```python
from build123d import *

# Parameters (mm, degrees)
CYLINDER049_R             = 1.38
CYLINDER049_DEPTH         = 40
CYLINDER030_R             = 1.75
CYLINDER030_DEPTH         = 10
CYLINDER029_R             = 5
CYLINDER029_DEPTH         = 10
CYLINDER024_R             = 8.5
CYLINDER024_DEPTH         = 2
BOX014_W                  = 0.5
BOX014_H                  = 1
BOX014_DEPTH              = 5
ARRAY002_COUNT            = 12
BOX015_W                  = 0.5
BOX015_H                  = 1
BOX015_DEPTH              = 5
CYLINDER026_R             = 4.5
CYLINDER026_DEPTH         = 8
CYLINDER028_R             = 1.5
CYLINDER028_DEPTH         = 4
BOX016_W                  = 1
BOX016_H                  = 10
BOX016_DEPTH              = 30
CYLINDER027_R             = 3
CYLINDER027_DEPTH         = 30
CYLINDER025_R             = 13
CYLINDER025_DEPTH         = 10
FUSION006_ROLL_ANGLE      = 180
FUSION006_PLACEMENT_ANGLE = 150
CYLINDER023_R             = 1.5
CYLINDER023_DEPTH         = 5
CYLINDER022_R             = 1.5
CYLINDER022_DEPTH         = 5
CYLINDER021_R             = 1.5
CYLINDER021_DEPTH         = 5
CYLINDER020_R             = 1.5
CYLINDER020_DEPTH         = 5
BOX010_W                  = 4
BOX010_H                  = 36
BOX010_DEPTH              = 38
BOX011_W                  = 4
BOX011_H                  = 36
BOX011_DEPTH              = 38
BOX012_W                  = 10
BOX012_H                  = 36
BOX012_DEPTH              = 3
BOX013_W                  = 10
BOX013_H                  = 36
BOX013_DEPTH              = 3
BOX009_W                  = 50
BOX009_H                  = 36
BOX009_DEPTH              = 3
CHAMFER_SIZE              = 2
CHAMFER001_SIZE           = 1


with BuildPart() as cylinder049:
    # Cylinder049 → Cylinder049 (new body)
    with BuildSketch(Plane(origin=(38, 57, 59), x_dir=(1, 0, 0), z_dir=(0, 0, 1))):
        Circle(CYLINDER049_R)
    extrude(amount=CYLINDER049_DEPTH)


with BuildPart() as cylinder030:
    # Cylinder030 → Cylinder030 (new body)
    with BuildSketch(Plane(origin=(33.25, 47.5, 71), x_dir=(1, 0, 0), z_dir=(0, 0, 1))):
        Circle(CYLINDER030_R)
    extrude(amount=CYLINDER030_DEPTH)


with BuildPart() as cylinder029:
    # Cylinder029 → Cylinder029 (new body)
    with BuildSketch(Plane(origin=(41, 43, 71), x_dir=(1, 0, 0), z_dir=(0, 0, 1))):
        Circle(CYLINDER029_R)
    extrude(amount=CYLINDER029_DEPTH)


with BuildPart() as cylinder024:
    # Cylinder024 → Cylinder024 (new body)
    with BuildSketch(Plane.XY.offset(10)):
        Circle(CYLINDER024_R)
    extrude(amount=CYLINDER024_DEPTH)


with BuildPart() as pin_array002:
    # Box014 → Box014 (new body)
    with BuildSketch(Plane(origin=(11, -0.5, -5), x_dir=(1, 0, 0), z_dir=(0, 0, 1))):
        with Locations((0.25, 0.5)):
            Rectangle(BOX014_W, BOX014_H)
    extrude(amount=BOX014_DEPTH)

    # Array002: Pin array002 ×12 about axis
    array002_axis = Axis((0, 0, 0), (0, 0, 1))


with BuildPart() as pin_array002_1:
    add(pin_array002.part)
    for i in range(1, ARRAY002_COUNT):
        add(pin_array002.part.rotate(array002_axis, i * 360 / ARRAY002_COUNT))


with BuildPart() as pin_central002:
    # Box015 → Box015 (new body)
    with BuildSketch(Plane(origin=(3, -0.5, -5), x_dir=(1, 0, 0), z_dir=(0, 0, 1))):
        with Locations((0.25, 0.5)):
            Rectangle(BOX015_W, BOX015_H)
    extrude(amount=BOX015_DEPTH)


with BuildPart() as cylinder026:
    # Cylinder026 → Cylinder026 (new body)
    with BuildSketch(Plane.XY.offset(12)):
        Circle(CYLINDER026_R)
    extrude(amount=CYLINDER026_DEPTH)


with BuildPart() as cylinder028:
    # Cylinder028 → Cylinder028 (new body)
    with BuildSketch(Plane(origin=(9, 0, 10), x_dir=(1, 0, 0), z_dir=(0, 0, 1))):
        Circle(CYLINDER028_R)
    extrude(amount=CYLINDER028_DEPTH)


with BuildPart() as obj1:
    # Box016 → Box016 (new body)
    with BuildSketch(Plane(origin=(2, -5, 20), x_dir=(1, 0, 0), z_dir=(0, 0, 1))):
        with Locations((0.5, 5)):
            Rectangle(BOX016_W, BOX016_H)
    extrude(amount=BOX016_DEPTH)


with BuildPart() as obj2:
    # Cylinder027 → Cylinder027 (new body)
    with BuildSketch(Plane.XY.offset(20)):
        Circle(CYLINDER027_R)
    extrude(amount=CYLINDER027_DEPTH)

    # Cut010: cut obj1
    add(obj1.part, mode=Mode.SUBTRACT)


with BuildPart() as selector_taladro:
    # Cylinder025 → Cylinder025 (new body)
    with BuildSketch(Plane.XY):
        Circle(CYLINDER025_R)
    extrude(amount=CYLINDER025_DEPTH)

    # Fusion006: union Cylinder024, Pin array002, Pin central002, Cylinder026, Cylinder028, obj2
    add(cylinder024.part)
    add(pin_array002_1.part)
    add(pin_central002.part)
    add(cylinder026.part)
    add(cylinder028.part)
    add(obj2.part)


with BuildPart() as selector_taladro_1:
    # Fusion006 roll: moved
    add(selector_taladro.part.rotate(Axis((0, 0, 0), (1, 0, 0)), FUSION006_ROLL_ANGLE))


with BuildPart() as selector_taladro_2:
    # Fusion006 placement: moved
    add(selector_taladro_1.part.moved(Location((40.992958, 43.010908, 90))).rotate(Axis((40.992958, 43.010908, 90), (0, 0, 1)), FUSION006_PLACEMENT_ANGLE))


with BuildPart() as cylinder023:
    # Cylinder023 → Cylinder023 (new body)
    with BuildSketch(Plane(origin=(65.5, 54, 39), x_dir=(1, 0, 0), z_dir=(0, 0, 1))):
        Circle(CYLINDER023_R)
    extrude(amount=CYLINDER023_DEPTH)


with BuildPart() as cylinder022:
    # Cylinder022 → Cylinder022 (new body)
    with BuildSketch(Plane(origin=(65.5, 38, 39), x_dir=(1, 0, 0), z_dir=(0, 0, 1))):
        Circle(CYLINDER022_R)
    extrude(amount=CYLINDER022_DEPTH)


with BuildPart() as cylinder021:
    # Cylinder021 → Cylinder021 (new body)
    with BuildSketch(Plane(origin=(8.5, 54, 39), x_dir=(1, 0, 0), z_dir=(0, 0, 1))):
        Circle(CYLINDER021_R)
    extrude(amount=CYLINDER021_DEPTH)


with BuildPart() as cylinder020:
    # Cylinder020 → Cylinder020 (new body)
    with BuildSketch(Plane(origin=(8.5, 38, 39), x_dir=(1, 0, 0), z_dir=(0, 0, 1))):
        Circle(CYLINDER020_R)
    extrude(amount=CYLINDER020_DEPTH)


with BuildPart() as box010:
    # Box010 → Box010 (new body)
    with BuildSketch(Plane(origin=(12, 28, 40), x_dir=(1, 0, 0), z_dir=(0, 0, 1))):
        with Locations((2, 18)):
            Rectangle(BOX010_W, BOX010_H)
    extrude(amount=BOX010_DEPTH)


with BuildPart() as box011:
    # Box011 → Box011 (new body)
    with BuildSketch(Plane(origin=(58, 28, 40), x_dir=(1, 0, 0), z_dir=(0, 0, 1))):
        with Locations((2, 18)):
            Rectangle(BOX011_W, BOX011_H)
    extrude(amount=BOX011_DEPTH)


with BuildPart() as box012:
    # Box012 → Box012 (new body)
    with BuildSketch(Plane(origin=(6, 28, 40), x_dir=(1, 0, 0), z_dir=(0, 0, 1))):
        with Locations((5, 18)):
            Rectangle(BOX012_W, BOX012_H)
    extrude(amount=BOX012_DEPTH)


with BuildPart() as box013:
    # Box013 → Box013 (new body)
    with BuildSketch(Plane(origin=(58, 28, 40), x_dir=(1, 0, 0), z_dir=(0, 0, 1))):
        with Locations((5, 18)):
            Rectangle(BOX013_W, BOX013_H)
    extrude(amount=BOX013_DEPTH)


with BuildPart() as cut028:
    # Box009 → Box009 (new body)
    with BuildSketch(Plane(origin=(12, 28, 75), x_dir=(1, 0, 0), z_dir=(0, 0, 1))):
        with Locations((25, 18)):
            Rectangle(BOX009_W, BOX009_H)
    extrude(amount=BOX009_DEPTH)

    # Fusion005: union Box010, Box011, Box012, Box013
    add(box010.part)
    add(box011.part)
    add(box012.part)
    add(box013.part)

    # Chamfer
    chamfer_edges = [cut028.edges().sort_by_distance(p)[0] for p in [
        (58, 46, 75),
        (16, 46, 75),
    ]]
    chamfer(chamfer_edges, length=CHAMFER_SIZE)

    # Chamfer001
    chamfer001_edges = [cut028.edges().sort_by_distance(p)[0] for p in [
        (62, 46, 43),
        (12, 46, 43),
    ]]
    chamfer(chamfer001_edges, length=CHAMFER001_SIZE)

    # Cut006: cut Cylinder020
    add(cylinder020.part, mode=Mode.SUBTRACT)

    # Cut007: cut Cylinder021
    add(cylinder021.part, mode=Mode.SUBTRACT)

    # Cut008: cut Cylinder022
    add(cylinder022.part, mode=Mode.SUBTRACT)

    # Cut009: cut Cylinder023
    add(cylinder023.part, mode=Mode.SUBTRACT)

    # Cut011: cut Selector taladro
    add(selector_taladro_2.part, mode=Mode.SUBTRACT)

    # Cut012: cut Cylinder029
    add(cylinder029.part, mode=Mode.SUBTRACT)

    # Cut013: cut Cylinder030
    add(cylinder030.part, mode=Mode.SUBTRACT)

    # Cut028: cut Cylinder049
    add(cylinder049.part, mode=Mode.SUBTRACT)


solid = cut028.part
```
CAD build for the part. Positions are in the model's coordinates, mm. A direction names the side the tool comes from. Coordinates: 2 decimals unless noted, no trailing zeros. Write each loop counter-clockwise with the first axis right and the second up, starting at its lowest first coordinate (ties: lowest second). Pieces come first, ordered by that corner, then holes.
(1) Cut at C-C, the plane y = 50.5. List the corners of the cut face in (x, z), and give its area (3 significant figures).
(2) Flat gauge pins, fed straight in: pin 1 (16.5 mm diameter, centred on y = 40, z = 60.5, fed in from -X); pin 2 (11 mm diameter, centred on x = 43, y = 49.5, fed in from -Z); pin 3 (4 mm diameter, centred on x = 65.5, y = 54, fed in from +Z). Where does each tip first touch, or does it go through?
(3) Cut at A-A, the plane x = 38. List the corners of the cut face in (y, z).
(4) Cut at D-D, the plane x = 65.5. List the corners of the cut face in (y, z).
(5) Two-plate mould, pull along X, no slides. Class faces 1 (the face through (62, 46, 61)), 2 (the face through (37, 46, 76)), 3 (the face through (37, 64, 76)), 4 (the face through (58, 46, 56)): +X half, -X half, draft (parallel to the pull), parting line (faces both ways), or undercut.
(6) Cut at B-B, the plane z = 64. List the corners of the cut face in (x, y), and give its area (3 significant figures).
(7) Drill centre lines: probe 1 along X at (y, z) = (38, 41.2); probe 2 along Y at (x, z) = (8.5, 41.2); probe 3 along Y at (x, z) = (41, 76). Where is each one in solid material? Low to high.
(8) 3-axis set-ups, long thin cutter, end or side, ignore diameter. For faces 5 (the face through (8, 46, 43)), 6 (the face through (32.87, 45.79, 76.48)), 7 (the face through (17, 46, 74)): which of +Z, -Z, +X, -X, +Y, -Y reach the whole face in a straight line?
Geometry says:
1. outline: (6, 40) - (16, 40) - (16, 73) - (18, 75) - (56, 75) - (58, 73) - (58, 40) - (68, 40) - (68, 43) - (63, 43) - (62, 44) - (62, 78) - (12, 78) - (12, 44) - (11, 43) - (6, 43) - close
1. area: 471 mm2
2. pin 1: stops at x = 12
2. pin 2: stops at z = 75
2. pin 3: stops at z = 43
3. outline: (28, 75) - (39, 75) - (39, 78) - (28, 78) - close; (47, 75) - (55.62, 75) - (55.62, 78) - (47, 78) - close; (58.38, 75) - (64, 75) - (64, 78) - (58.38, 78) - close
4. outline: (28, 40) - (36.5, 40) - (36.5, 43) - (28, 43) - close; (39.5, 40) - (52.5, 40) - (52.5, 43) - (39.5, 43) - close; (55.5, 40) - (64, 40) - (64, 43) - (55.5, 43) - close
5. face 1: +X half
5. face 2: undercut
5. face 3: draft
5. face 4: undercut
6. outline: (12, 28) - (16, 28) - (16, 64) - (12, 64) - close; (58, 28) - (62, 28) - (62, 64) - (58, 64) - close
6. area: 288 mm2
7. probe 1: x = 6 to 7, 10 to 16, 58 to 64, 67 to 68
7. probe 2: y = 28 to 36.5, 39.5 to 52.5, 55.5 to 64
7. probe 3: y = 28 to 38, 48 to 64
8. face 5: +Z, -X, +Y, -Y
8. face 6: +Z, -Z
8. face 7: -Z, +Y, -Y
